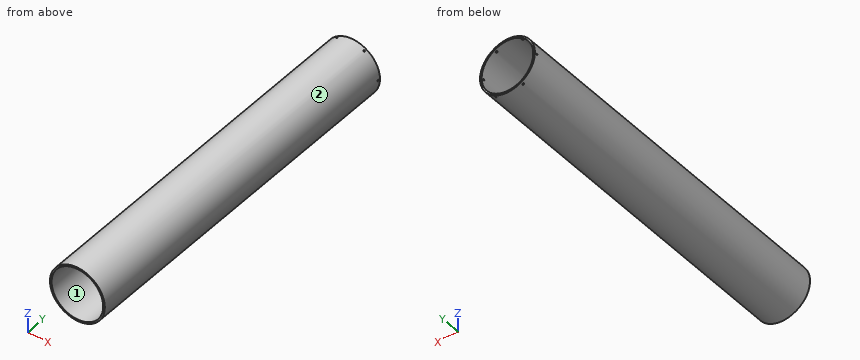
from build123d import *

# Parameters (mm, degrees)
SKETCH1_R           = 53.975
SKETCH1_R_2         = 50.8
BOSS_EXTRUDE1_DEPTH = 711.2
SKETCH2_R           = 1.5875
CUT_EXTRUDE1_DEPTH  = 54.975
CIRPATTERN1_COUNT   = 3


with BuildPart() as part:
    # Sketch1 → Boss-Extrude1 (new body)
    with BuildSketch(Plane(origin=(0, 0, 0), x_dir=(1, 0, 0), z_dir=(0, 1, 0))):
        Circle(SKETCH1_R)
        Circle(SKETCH1_R_2, mode=Mode.SUBTRACT)
    extrude(amount=BOSS_EXTRUDE1_DEPTH)

    # Sketch2 → Cut-Extrude1 (cut, symmetric)
    with BuildSketch(Plane(origin=(0, 0, 0), x_dir=(0, 0, -1), z_dir=(1, 0, 0))):
        with Locations((0, 705.84695)):
            Circle(SKETCH2_R)
    cut_extrude1 = extrude(amount=CUT_EXTRUDE1_DEPTH, both=True, mode=Mode.SUBTRACT)

    # CirPattern1: Cut-Extrude1 ×3 about axis
    cirpattern1_axis = Axis((0, 711.2, 0), (0, 1, 0))
    for i in range(1, CIRPATTERN1_COUNT):
        add(cut_extrude1.rotate(cirpattern1_axis, i * 360 / CIRPATTERN1_COUNT), mode=Mode.SUBTRACT)


solid = part.part
Design review of the part built by this model. Coordinates are the model's own, in mm. Face numbers are marked on the shaded views. Coordinates: 2 decimals unless noted, no trailing zeros. Loops run counter-clockwise (first coordinate to the right, second up) from the corner with the lowest first, then second, coordinate; pieces in that order, holes last. Notation, with made-up numbers: (32.5, 33.5) -> (52.5, 33.5) arc R13 cw to (52.5, 56.5) -> close; hole circle Ø2 at (9.25, -24). An arc over 180 degrees is marked (long way). Use a Markdown table: item, result. Add a question column.
Item 1: We need section B-B, the plane z = -24.5. Write out the cut boundary in (x, y), and give its area (3 significant figures).
Item 2: The part is to be moulded in two halves that separate along X. For the marked faces 1 and 2, say which applies: +X half, -X half, draft (parallel to the pull), parting line (faces both ways), or undercut.
Item 3: Wall thickness on L1, parallel to Z at x = 1, y = 599; L2, parallel to Y at x = -53.3, z = 0; L3, parallel to X at y = 412, z = 0 (3 decimals): over which ranges is each line inside the solid? List them lowest first. Write a range as from..to.
Item 4: We need section A-A, the plane x = 0. Write out the cut boundary in (y, z) (3 decimals), and give its area (3 significant figures).
Item 5: Clearance check with flat-ended pins moving along their axes: P1, Ø2, axis at y = 455, z = -32, coming from the +X side; P2, Ø10, axis at x = -17.5, y = 108.5, coming from the +Z side; P3, Ø12, axis at y = 242.5, z = -30, coming from the +X side. State where each tip first meets the part, or that it passes through.
Item 6: We need section C-C, the plane y = 438.5. Write out the cut boundary in (x, z) (3 decimals), and give its area (3 significant figures).
Numbers:
| question | item | result |
|---|---|---|
| 1 | outline | (-48.09, 0) -> (-44.5, 0) -> (-44.5, 711.2) -> (-48.09, 711.2) -> close; (44.5, 0) -> (48.09, 0) -> (48.09, 711.2) -> (44.5, 711.2) -> close |
| 1 | area | 5,110 mm^2 |
| 2 | face 1 | undercut |
| 2 | face 2 | parting line |
| 3 | L1 | z = -53.97..-50.79, 50.79..53.97 |
| 3 | L2 | y = 0..704.26, 707.43..711.2 |
| 3 | L3 | x = -53.975..-50.8, 50.8..53.975 |
| 4 | outline | (0, -53.975) -> (711.2, -53.975) -> (711.2, -50.8) -> (0, -50.8) -> close; (0, 50.8) -> (711.2, 50.8) -> (711.2, 53.975) -> (0, 53.975) -> close |
| 4 | area | 4,520 mm^2 |
| 5 | P1 | stops at x = 44.18 |
| 5 | P2 | stops at z = 52.51 |
| 5 | P3 | stops at x = 48.35 |
| 6 | outline | circle Ø107.95 at (0, 0); hole circle Ø101.6 at (0, 0) |
| 6 | area | 1,050 mm^2 |
